```python
from build123d import *

# Parameters (mm, degrees)
SKETCH1_R           = 27.5
SKETCH1_R_2         = 3
BOSS_EXTRUDE1_DEPTH = 10
SKETCH2_R           = 15
BOSS_EXTRUDE2_DEPTH = 10
SKETCH3_R           = 8
BOSS_EXTRUDE3_DEPTH = 150


with BuildPart() as part:
    # Sketch1 → Boss-Extrude1 (new body)
    with BuildSketch(Plane.XY):
        Circle(SKETCH1_R)
        with Locations((0, 20)):
            Circle(SKETCH1_R_2, mode=Mode.SUBTRACT)
        with Locations((17.320508076, -10)):
            Circle(SKETCH1_R_2, mode=Mode.SUBTRACT)
        with Locations((-17.320508076, -10)):
            Circle(SKETCH1_R_2, mode=Mode.SUBTRACT)
    extrude(amount=BOSS_EXTRUDE1_DEPTH)

    # Sketch2 → Boss-Extrude2 (add)
    with BuildSketch(Plane.XY.offset(10)):
        Circle(SKETCH2_R)
    extrude(amount=BOSS_EXTRUDE2_DEPTH)

    # Sketch3 → Boss-Extrude3 (add)
    with BuildSketch(Plane.XY.offset(20)):
        Circle(SKETCH3_R)
    extrude(amount=BOSS_EXTRUDE3_DEPTH)


solid = part.part
```
The model under review builds one solid part; all positions refer to its coordinate system, in mm. A direction names the side the tool comes from. Round coordinates to 2 decimals unless told otherwise and drop trailing zeros. Write each loop counter-clockwise with the first axis right and the second up, starting at its lowest first coordinate (ties: lowest second). Pieces come first, ordered by that corner, then holes. Notation, with made-up numbers: (-32.5, 88.5) -> (5.5, 88.5) arc R21 ccw to (5.5, 123.5) -> close; hole circle Ø2 at (-2, 21.5). An arc over 180 degrees is marked (long way). Use CSV: the item, a comma, the result in double quotes.
Q1. To check wall thickness, follow probe 1 along Y at (x, z) = (0, 3.5); probe 2 along Z at (x, y) = (-16.5, 4.5); probe 3 along Z at (x, y) = (-5, 9). State the ranges of each line that lie inside material, in increasing order. Write a range as [from, to].
Checks:
probe 1,"[-27.5, 17], [23, 27.5]"
probe 2,"[0, 10]"
probe 3,"[0, 20]"
Q2. Consider section A-A (x = 0). Give the boundary of the cut face in (y, z).
Checks:
outline,"(-27.5, 0) -> (17, 0) -> (17, 10) -> (15, 10) -> (15, 20) -> (8, 20) -> (8, 170) -> (-8, 170) -> (-8, 20) -> (-15, 20) -> (-15, 10) -> (-27.5, 10) -> close; (23, 0) -> (27.5, 0) -> (27.5, 10) -> (23, 10) -> close"
Q3. Consider section C-C (y = 0). Give the boundary of the cut face in (x, z), then the cut area to 3 significant figures.
Checks:
outline,"(-27.5, 0) -> (27.5, 0) -> (27.5, 10) -> (15, 10) -> (15, 20) -> (8, 20) -> (8, 170) -> (-8, 170) -> (-8, 20) -> (-15, 20) -> (-15, 10) -> (-27.5, 10) -> close"
area,"3,250 mm²"
Q4. For pin 1 Ø7 at (x, y) = (0, 20) entering from +Z; pin 2 Ø8 at (x, y) = (-14.5, 3) entering from +Z; pin 3 Ø1.5 at (y, z) = (4.5, 84.5) entering from +X, all flat-tipped, find the tip position at first contact; note any pin that passes through.
Checks:
pin 1,"z = 10"
pin 2,"z = 20"
pin 3,"x = 7.07"
Q5. Consider section B-B (y = -10). Give the boundary of the cut face in (x, z), then the cut area to 3 significant figures.
Checks:
outline,"(-25.62, 0) -> (-20.32, 0) -> (-20.32, 10) -> (-25.62, 10) -> close; (-14.32, 0) -> (14.32, 0) -> (14.32, 10) -> (11.18, 10) -> (11.18, 20) -> (-11.18, 20) -> (-11.18, 10) -> (-14.32, 10) -> close; (20.32, 0) -> (25.62, 0) -> (25.62, 10) -> (20.32, 10) -> close"
area,"616 mm²"
Q6. For faces 1 (the flat face through (6, -6, 20)), 2 (the flat face through (0, 0, 170)), list the 3-axis set-ups (+Z, -Z, +X, -X, +Y, -Y) from which the entire face can be reached by the end or side of a thin tool; tool diameter is ignored.
Checks:
face 1,"+Z"
face 2,"+Z, +X, -X, +Y, -Y"
Q7. Consider section D-D (z = 79). Give the boundary of the cut face in (x, y), then the cut area to 3 significant figures.
Checks:
outline,"circle Ø16 at (0, 0)"
area,"201 mm²"
Q8. Mouldability with a two-part tool opening along X and no side actions: class faces 3 (the cylindrical face through (-5.961, -26.846, 4.93)), 4 (the cylindrical face through (16.93, -7.026, 4.93)), 5 (the flat face through (0, 0, 0)) as released by +X, released by -X, zero draft, split by the parting line, or undercut.
Checks:
face 3,"split by the parting line"
face 4,"undercut"
face 5,"zero draft"
